Autodesk Inventor part; units mm, degrees
ref_plane "YZ Plane" through (0, 0, 0) normal (1, 0, 0) x (0, 1, 0)
ref_plane "XZ Plane" through (0, 0, 0) normal (0, 1, 0) x (-1, 0, 0)
ref_plane "XY Plane" through (0, 0, 0) normal (0, 0, 1) x (1, 0, 0)
sketch "Sketch1" plane through (0, 0, 0) normal (0, 0, 1) x (1, 0, 0)
  line L0 (0, 0) -> (539.75, 0)
  line L1 (539.75, 0) -> (539.75, 603.25)
  line L2 (539.75, 603.25) -> (0, 603.25)
  line L3 (0, 603.25) -> (0, 0)
  line L4 (174.625, 603.25) -> (365.125, 603.25)
  line L5 (365.125, 603.25) -> (365.125, 563.25)
  line L6 (365.125, 563.25) -> (174.625, 563.25)
  line L7 (174.625, 563.25) -> (174.625, 603.25)
  point P0 (269.875, 603.25)
  dimension "d0" = 603.25
  dimension "d1" = 539.75
  dimension "d4" = 40
  dimension "d5" = 190.5
extrude "Extrusion1" add sketch "Sketch1" along normal blind 6.35 contours L3 L2 L7 L6 L5 L1 L0
hole "Hole1" at (463.55, 527.05, 0) direction (0, 0, 1) diameter 4.4958 end through all
hole "Hole2" at (404.876, 527.05, 0) direction (0, 0, 1) diameter 4.4958 end through all
sketch "Sketch2" plane through (0, 0, 0) normal (0, 0, -1) x (-1, 0, 0)
  line L0 (-539.75, 603.25) -> (-365.125, 603.25)
  line L1 (-539.75, 0) -> (-539.75, 603.25)
  line L2 (-174.625, 563.25) -> (-365.125, 563.25)
  line L3 (-488.95, 463.55) -> (-400.05, 463.55)
  point P0 (-444.5, 463.55)
  dimension "d24" = 88.9
  dimension "d25" = 50.8
  dimension "d27" = 139.7
hole "Hole3" at (488.95, 463.55, 0) at (400.05, 463.55, 0) direction (0, 0, 1) diameter 3.81 end through all
hole "Hole4" at (463.55, 254, 0) direction (0, 0, 1) diameter 6.7564 end through all
hole "Hole5" at (436.88, 197.358, 0) direction (0, 0, 1) diameter 6.7564 end through all
sketch "Sketch3" plane through (0, 0, 0) normal (0, 0, -1) x (-1, 0, 0)
  circle A0 centre (-436.88, 197.358) radius 3.3782
  circle A1 centre (-463.55, 254) radius 3.3782
  point P0 (-436.88, 292.1)
  point P1 (-463.55, 158.75)
  dimension "d53" = 133.35
  dimension "d54" = 38.1
hole "Hole6" at (436.88, 292.1, 0) at (463.55, 158.75, 0) direction (0, 0, 1) diameter 15.875 end through all
properties part number "top plate" material "Polycarbonate, Clear"
Can you work these out from the model? Positions are in its coordinate system, mm. Coordinates: 2 decimals unless noted, no trailing zeros. Loops run counter-clockwise (first coordinate to the right, second up) from the corner with the lowest first, then second, coordinate; pieces in that order, holes last.
1) Thinking about a two-plate mould opening in X: for faces 1 (the flat face through (266, 306, 6.35)), 2 (the cylindrical face through (456.86, 163.02, 3.22)), 3 (the cylindrical face through (444.63, 290.38, 3.22)), which applies, pulls with the +X half, pulls with the -X half, needs draft (parallel to the pull), parting line crosses it, or undercut?
2) Imagine slicing it at B-B on z = 2. State how many separate pieces and enclosed holes the cut face has, plus the area to 3 significant figures.
3) Imagine slicing it at A-A on y = 158.75. List the corners of the cut face in (x, z) for me.
4) For pin 1 (5.5 mm diameter, centred on x = 463.55, y = 254, fed in from +Z); pin 2 (1.9 mm diameter, centred on x = 303, z = 3, fed in from +Y), each with a flat end and sliding along its axis, tell me the tip position at first contact or that it passes through.
5) Imagine slicing it at C-C on x = 326.5. List the corners of the cut face in (y, z) for me.
6) I need wall thicknesses on probe 1 along X at (y, z) = (463.55, 5) (3 decimals); probe 2 along Y at (x, z) = (463.55, 4); probe 3 along X at (y, z) = (254, 1.5). Which ranges of each line are inside material? Lowest first, please.
Completed:
1. face 1: needs draft
1. face 2: undercut
1. face 3: undercut
2. separate pieces: 1
2. enclosed holes: 8
2. area: 317,000 mm2
3. outline: (0, 0) - (455.61, 0) - (455.61, 6.35) - (0, 6.35) - close; (471.49, 0) - (539.75, 0) - (539.75, 6.35) - (471.49, 6.35) - close
4. pin 1: passes through
4. pin 2: stops at y = 563.25
5. outline: (0, 0) - (563.25, 0) - (563.25, 6.35) - (0, 6.35) - close
6. probe 1: x = 0 to 398.145, 401.955 to 487.045, 490.855 to 539.75
6. probe 2: y = 0 to 150.81, 166.69 to 250.62, 257.38 to 524.8, 529.3 to 603.25
6. probe 3: x = 0 to 460.17, 466.93 to 539.75
